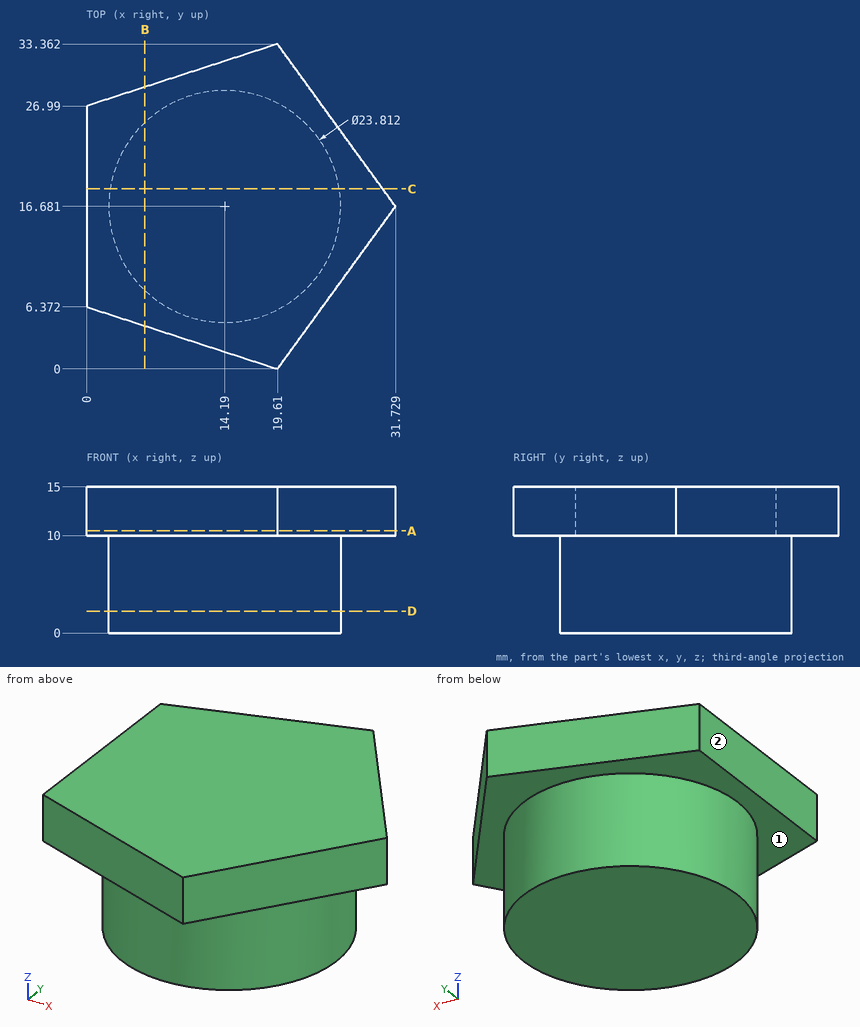
Study the drawing (mm; zero at the part's minimum x, y, z) and answer. A direction names the side the tool comes from. Give positions to 0.01 mm unless a question says otherwise; leave off trailing zeros. Order: outer loops, then holes, each group sorted by start corner. A loop starts at its lowest first (then second) coordinate and runs counter-clockwise, first axis right, second up. Notation, with made-up numbers: (81, 59.25) -> (127, 59.25) arc R28 ccw to (127, 90.25) -> close; hole circle Ø2 at (-5, 5). An arc over 180 degrees is marked (long way). Write item = value, one per line.
1. For the marked faces 1 and 2, determine the directions among +Z, -Z, +X, -X, +Y, -Y from which every point of the face is accessible in a straight line to the end or side of a thin tool.
Numbers:
face_1 = -Z
face_2 = +Z, -Z, -X, +Y, -Y
2. Straight lines are drawn through the part: line 1 along Z through (x, y) = (17.5, 31); line 2 along X through (y, z) = (10, 12.5) (1 decimal); line 3 along X through (y, z) = (24, 14.75). For each, find the intervals that lie inside material, in ascending order.
Numbers:
line_1 = 10 to 15
line_2 = 0 to 26.9
line_3 = 0 to 26.41
3. A cutting plane is placed at D-D, the plane z = 2.25. Write down the section's boundary in (x, y) (1 decimal), and give its area (3 significant figures).
Numbers:
outline = circle Ø23.8 at (14.2, 16.7)
area = 445 mm²
4. A cutting plane is placed at A-A, the plane z = 10.5. Write down the section's boundary in (x, y).
Numbers:
outline = (0, 6.37) -> (19.61, 0) -> (31.73, 16.68) -> (19.61, 33.36) -> (0, 26.99) -> close
5. A cutting plane is placed at C-C, the plane y = 18.5. Write down the section's boundary in (x, z) (1 decimal).
Numbers:
outline = (0, 10) -> (2.4, 10) -> (2.4, 0) -> (26, 0) -> (26, 10) -> (30.4, 10) -> (30.4, 15) -> (0, 15) -> close
6. Given pin 1 (6 mm diameter, centred on y = 12.5, z = 9, fed in from +X) (1 decimal); pin 2 (5 mm diameter, centred on x = 6.5, z = 4, fed in from -Y) (1 decimal); pin 3 (2 mm diameter, centred on y = 18, z = 6.5, fed in from +X), each flat-ended and moving along its own axis, determine where each tip first touches the part or whether it passes through.
Numbers:
pin_1 = 30.7
pin_2 = 6
pin_3 = 26.09
7. A cutting plane is placed at B-B, the plane x = 6. Write down the section's boundary in (y, z), and give its area (3 significant figures).
Numbers:
outline = (4.42, 10) -> (8.04, 10) -> (8.04, 0) -> (25.32, 0) -> (25.32, 10) -> (28.94, 10) -> (28.94, 15) -> (4.42, 15) -> close
area = 295 mm²
